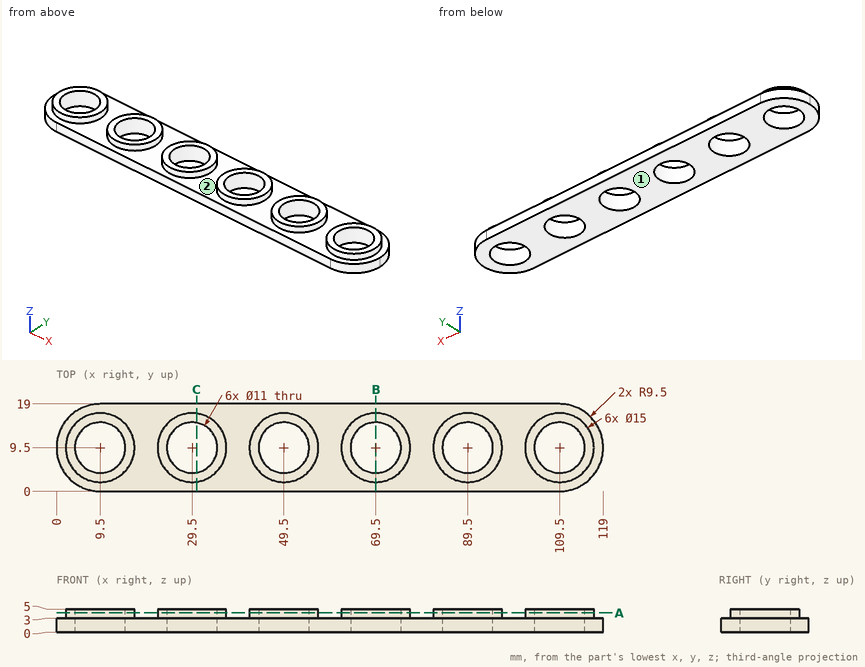
Verification items for this drawing (mm, ordinates from the low corner). Give positions to 0.01 mm unless a question says otherwise; leave off trailing zeros. Write each loop counter-clockwise with the first axis right and the second up, starting at its lowest first coordinate (ties: lowest second). Pieces come first, ordered by that corner, then holes. Notation, with made-up numbers: (17.5, -10.5) -> (43.5, -10.5) arc R29 ccw to (43.5, 10.5) -> close; hole circle Ø3 at (-22.75, 87). An arc over 180 degrees is marked (long way). Use one line per item in the form item = value.
Item 1: Sectioned sample at B-B on x = 69.5. Enter the section's corners in (y, z).
Results list:
outline = (0, 0) -> (4, 0) -> (4, 5) -> (2, 5) -> (2, 3) -> (0, 3) -> close; (15, 0) -> (19, 0) -> (19, 3) -> (17, 3) -> (17, 5) -> (15, 5) -> close
Item 2: Sectioned sample at A-A on z = 4.2. Count the separate pieces of the cut face and the enclosed holes in it, plus the area to 3 significant figures.
Results list:
separate_pieces = 6
enclosed_holes = 6
area = 490 mm2
Item 3: Mould release check, pull along X, two halves, no side actions. Record for the marked faces 1 and 2: released by +X, released by -X, zero draft, split by the parting line, or undercut.
Results list:
face_1 = zero draft
face_2 = undercut
Item 4: Depth check by flat-ended pin: pin 1 Ø5 at (x, y) = (20.5, 3) entering from +Z; pin 2 Ø1.5 at (y, z) = (5.5, 2) entering from -X; pin 3 Ø3 at (y, z) = (4.5, 3.5) entering from +X. Enter the tip coordinate at first touch or a pass-through.
Results list:
pin_1 = 3
pin_2 = 0.57
pin_3 = 118.3
Item 5: Sectioned sample at C-C on x = 30.5. Enter the section's corners in (y, z).
Results list:
outline = (0, 0) -> (4.09, 0) -> (4.09, 5) -> (2.07, 5) -> (2.07, 3) -> (0, 3) -> close; (14.91, 0) -> (19, 0) -> (19, 3) -> (16.93, 3) -> (16.93, 5) -> (14.91, 5) -> close
Item 6: Scan lines: line 1 (Y direction, x = 69.5, z = 2.2); line 2 (Z direction, x = 39.5, y = 12.5); line 3 (Y direction, x = 94, z = 3.5). Record each from-to range of solid material in increasing order.
Results list:
line_1 = 0 to 4, 15 to 19
line_2 = 0 to 3
line_3 = 3.5 to 6.34, 12.66 to 15.5
